Geometry: final body of the model. Coordinates: model frame, mm. Face numbers are marked on the shaded views. Coordinates: 2 decimals unless noted, no trailing zeros. Write each loop counter-clockwise with the first axis right and the second up, starting at its lowest first coordinate (ties: lowest second). Pieces come first, ordered by that corner, then holes.
from build123d import *

# Parameters (mm, degrees)
SKETCH2_R           = 115
BOSS_EXTRUDE1_DEPTH = 20
SKETCH3_R           = 112
BOSS_EXTRUDE5_DEPTH = 5
SKETCH6_R           = 109
CUT_EXTRUDE2_DEPTH  = 22
SKETCH9_W           = 58
SKETCH9_H           = 90
BOSS_EXTRUDE9_DEPTH = 5
SKETCH10_W          = 52
SKETCH10_H          = 86
CUT_EXTRUDE3_DEPTH  = 5
CUT_EXTRUDE4_DEPTH  = 165.544826719
SKETCH13_R          = 3
CUT_EXTRUDE5_DEPTH  = 165.544826874


with BuildPart() as part:
    # Sketch2 → Boss-Extrude1 (new body)
    with BuildSketch(Plane(origin=(0, 0, 0), x_dir=(1, 0, 0), z_dir=(0, 1, 0))):
        with Locations(Location((0, 0, 0), (0, 0, 270))):
            Circle(SKETCH2_R)
    extrude(amount=BOSS_EXTRUDE1_DEPTH)

    # Sketch3 → Boss-Extrude5 (add)
    with BuildSketch(Plane(origin=(0, 20, 0), x_dir=(1, 0, 0), z_dir=(0, 1, 0))):
        with Locations(Location((0, 0, 0), (0, 0, 270))):
            Circle(SKETCH3_R)
    extrude(amount=BOSS_EXTRUDE5_DEPTH)

    # Sketch6 → Cut-Extrude2 (cut)
    with BuildSketch(Plane(origin=(0, 25, 0), x_dir=(1, 0, 0), z_dir=(0, 1, 0))):
        with Locations(Location((0, 0, 0), (0, 0, 270))):
            Circle(SKETCH6_R)
    extrude(amount=-CUT_EXTRUDE2_DEPTH, mode=Mode.SUBTRACT)

    # Sketch9 → Boss-Extrude9 (add)
    with BuildSketch(Plane(origin=(0, 3, 0), x_dir=(1, 0, 0), z_dir=(0, 1, 0))):
        with Locations((0, -59)):
            Rectangle(SKETCH9_W, SKETCH9_H)
    extrude(amount=BOSS_EXTRUDE9_DEPTH)

    # Sketch10 → Cut-Extrude3 (cut)
    with BuildSketch(Plane(origin=(0, 8, 0), x_dir=(1, 0, 0), z_dir=(0, 1, 0))):
        with Locations((0, -61)):
            Rectangle(SKETCH10_W, SKETCH10_H)
    extrude(amount=-CUT_EXTRUDE3_DEPTH, mode=Mode.SUBTRACT)

    # Sketch12 → Cut-Extrude4 (cut, through all)
    with BuildSketch(Plane.XY):
        with BuildLine():
            Line((-3.5, 17.5), (3.5, 17.5))
            ThreePointArc((3.5, 17.5), (7, 14), (3.5, 10.5))
            Line((3.5, 10.5), (-3.5, 10.5))
            ThreePointArc((-3.5, 10.5), (-7, 14), (-3.5, 17.5))
        make_face()
    extrude(amount=CUT_EXTRUDE4_DEPTH, mode=Mode.SUBTRACT)

    # Sketch13 → Cut-Extrude5 (cut, through all)
    with BuildSketch(Plane.XY):
        with Locations(Location((20, 14, 0), (0, 0, 180))):
            Circle(SKETCH13_R)
    extrude(amount=CUT_EXTRUDE5_DEPTH, mode=Mode.SUBTRACT)


solid = part.part
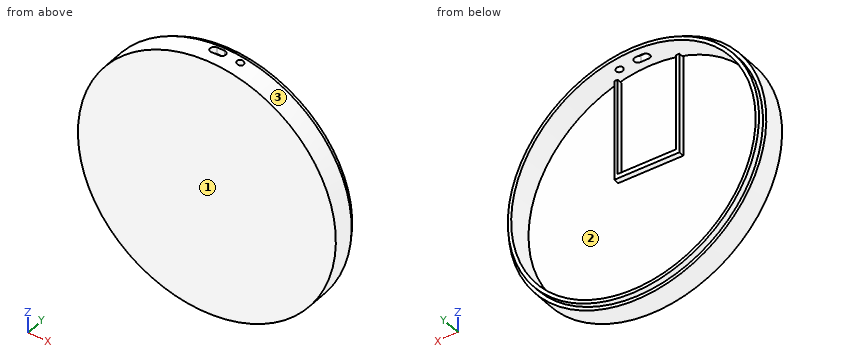
Item 1: Pull-direction query (X, two-part tool) for the marked faces 1, 2 and 3; classes: released by +X, released by -X, zero draft, split by the parting line, or undercut.
Derived:
face 1: zero draft
face 2: undercut
face 3: split by the parting line
Item 2: Section B-B, the plane z = 0. Output: boundary loops of the cut face in (x, y), plus the area to 3 significant figures.
Derived:
outline: (-115, 0) - (115, 0) - (115, 20) - (112, 20) - (112, 25) - (109, 25) - (109, 3) - (-109, 3) - (-109, 25) - (-112, 25) - (-112, 20) - (-115, 20) - close
area: 924 mm2
Item 3: Section D-D, the plane z = 100. Output: boundary loops of the cut face in (x, y).
Derived:
outline: (-56.79, 0) - (56.79, 0) - (56.79, 20) - (50.44, 20) - (50.44, 25) - (43.37, 25) - (43.37, 3) - (29, 3) - (29, 8) - (26, 8) - (26, 3) - (-26, 3) - (-26, 8) - (-29, 8) - (-29, 3) - (-43.37, 3) - (-43.37, 25) - (-50.44, 25) - (-50.44, 20) - (-56.79, 20) - close
Item 4: Section A-A, the plane x = 0. Output: boundary loops of the cut face in (y, z), plus the area to 3 significant figures.
Derived:
outline: (0, -115) - (20, -115) - (20, -112) - (25, -112) - (25, -109) - (3, -109) - (3, 14) - (8, 14) - (8, 18) - (3, 18) - (3, 109) - (10.5, 109) - (10.5, 115) - (0, 115) - close; (17.5, 109) - (25, 109) - (25, 112) - (20, 112) - (20, 115) - (17.5, 115) - close
area: 902 mm2
Item 5: Material intervals for probe 1 along X at (y, z) = (11, -1); probe 2 along X at (y, z) = (20.75, 0); probe 3 along Y at (x, z) = (-61, 79.5), sorted ascending.
Derived:
probe 1: x = -115 to -109, 109 to 115
probe 2: x = -112 to -109, 109 to 112
probe 3: y = 0 to 3
Item 6: Section C-C, the plane x = 68. Output: boundary loops of the cut face in (y, z), plus the area to 3 significant figures.
Derived:
outline: (0, -92.74) - (20, -92.74) - (20, -88.99) - (25, -88.99) - (25, -85.19) - (3, -85.19) - (3, 85.19) - (25, 85.19) - (25, 88.99) - (20, 88.99) - (20, 92.74) - (0, 92.74) - close
area: 851 mm2
Item 7: Pin query (flat end, axial travel): pin 1 (6 mm diameter, centred on x = -57, z = 6.5, fed in from +Y); pin 2 (3 mm diameter, centred on y = 4, z = 18.5, fed in from -X); pin 3 (5.5 mm diameter, centred on x = 8.5, y = 5, fed in from +Z). Return the tip coordinate at first contact, or that it passes through.
Derived:
pin 1: stops at y = 3
pin 2: stops at x = -113.74
pin 3: stops at z = 114.86
